Source: CAD feature listing. Evaluate the final solid. Frame: model axes, mm. A direction names the side the tool comes from. Coordinates: 2 decimals unless noted, no trailing zeros. Order: outer loops, then holes, each group sorted by start corner. A loop starts at its lowest first (then second) coordinate and runs counter-clockwise, first axis right, second up.
Autodesk Inventor part; units mm, degrees
ref_plane "Start plane" through (0, 0, 0) normal (0, 0, 1) x (1, 0, 0)
ref_plane "End plane" through (0, 0, 1) normal (0, 0, 1) x (1, 0, 0)
ref_plane "YZ Plane" through (0, 0, 0) normal (1, 0, 0) x (0, 1, 0)
ref_plane "Start plane" through (0, 0, 0) normal (0, 0, 1) x (1, 0, 0)
ref_plane "End plane" through (0, 0, 1) normal (0, 0, 1) x (1, 0, 0)
sketch "Sketch2" plane through (0, 0, 0) normal (0, 0, 1) x (1, 0, 0)
  line L0 (-2.02, 18.1) -> (-2.02, -2.9)
  line L1 (-5.02, 20.1) -> (-4.02, 20.1)
  line L2 (-5.02, -9.9) -> (-5.02, 20.1)
  line L3 (14.98, -9.9) -> (-5.02, -9.9)
  line L4 (14.98, -8.9) -> (14.98, -9.9)
  line L5 (1.98, -6.9) -> (12.98, -6.9)
  arc A0 (-2.02, -2.9) -> (1.98, -6.9) centre (1.98, -2.9) ccw
  arc A1 (-2.02, 18.1) -> (-4.02, 20.1) centre (-4.02, 18.1) ccw
  arc A2 (14.98, -8.9) -> (12.98, -6.9) centre (12.98, -8.9) ccw
  line L6 (0, 26.5971) -> (0, -15.9828) construction
  line L7 (-9.1028, 0) -> (19.4771, 0) construction
  point P0 (-2.02, 20.1)
  point P1 (-2.02, -6.9)
  point P2 (14.98, -6.9)
  dimension "d4" = 20
  dimension "d6" = 30
  dimension "d8" = 3
  dimension "d10" = 3
  dimension "d17" = 4
  dimension "d18" = 2
  dimension "d19" = 9.9
  dimension "d20" = 5.02
extrude "Body" add sketch "Sketch2" along normal blind 500 from surface at 0
sketch "Sketch3" plane through (0, 0, 0) normal (0, 0, 1) x (1, 0, 0)
  line L0 (0, 0) -> (10, 0)
ref_plane "Work Plane10" through (0, 0, 0) normal (0, -1, 0) x (1, 0, 0)
sketch "Sketch4" plane through (0, 0, 0) normal (0, -1, 0) x (1, 0, 0)
  line L0 (-2, 0) -> (12, 0)
  line L1 (-2, 1) -> (12, 1)
  dimension "d24" = 1
equation "\"d4\" = b"
equation "\"d6\" = ParH"
equation "\"d17\" = R"
equation "\"d18\" = R1"
equation "\"d19\" = ex"
equation "\"d20\" = ey"
equation "\"b\" = 20"
equation "\"ParT\" = 3"
equation "\"R1\" = 2"
equation "\"G_L\" = d24"
equation "\"ParH\" = 30"
equation "\"R\" = 4"
equation "\"ey\" = 5.02"
equation "\"ex\" = 9.9"
equation "\"G_OFFSET_START\" = 0"
equation "\"G_OFFSET_END\" = 0"
equation "\"d22\" = G_OFFSET_END + B_L"
equation "\"B_L\" = 1"
properties part number "ISO 657-2 - 30x 20x 3-1" material "Steel, Mild"
1. Section query B-B on x = 5. Return loops of the section in (y, z), plus the area to 3 significant figures.
Findings:
outline: (-9.9, 0) - (-6.9, 0) - (-6.9, 500) - (-9.9, 500) - close
area: 1,500 mm2
2. Access query for faces 1 (the face through (-2.02, 8, 246)), 2 (the face through (-2.5, 0.7, 0)). Directions: +Z, -Z, +X, -X, +Y, -Y. A direction counts if a zero-diameter tool reaches every point of the face in a straight line with its end or side. Return the directions, or none.
Findings:
face 1: +Z, -Z, +X, +Y
face 2: -Z, +X, -X, +Y, -Y
3. Ray query, line 1 (X direction, y = 2, z = 466); line 2 (Y direction, x = 8.25, z = 434); line 3 (Y direction, x = -3.75, z = 91). Return the intervals inside material, ascending.
Findings:
line 1: x = -5.02 to -2.02
line 2: y = -9.9 to -6.9
line 3: y = -9.9 to 20.08
4. Section query C-C on y = 11.75. Return loops of the section in (x, z).
Findings:
outline: (-5.02, 0) - (-2.02, 0) - (-2.02, 500) - (-5.02, 500) - close
5. Pin query (flat end, axial travel): P1, Ø9, axis at x = 5, z = 272.5, coming from the +Y side; P2, Ø6.5, axis at y = 4.5, z = 324.5, coming from the +X side; P3, Ø4, axis at x = 7, z = 75.5, coming from the +Y side. Return the tip coordinate at first contact, or that it passes through.
Findings:
P1: stops at y = -6.62
P2: stops at x = -2.02
P3: stops at y = -6.9
6. Section query A-A on z = 78. Return loops of the section in (x, y), plus the area to 3 significant figures.
Findings:
outline: (-5.02, -9.9) - (14.98, -9.9) - (14.98, -8.9) arc R2 ccw to (12.98, -6.9) - (1.98, -6.9) arc R4 cw to (-2.02, -2.9) - (-2.02, 18.1) arc R2 ccw to (-4.02, 20.1) - (-5.02, 20.1) - close
area: 143 mm2
